Here's how the part is built. I have some questions about the finished solid (model axes, mm). Coordinates: 2 decimals unless noted, no trailing zeros.
```python
from build123d import *

# Parameters (mm, degrees)
BOSS_EXTRUDE1_DEPTH  = 2
CUT_EXTRUDE8_DEPTH   = 3
SKETCH3_R            = 2.15
CUT_EXTRUDE9_DEPTH   = 3
SKETCH4_R            = 12
SKETCH4_R_2          = 1.65
CUT_EXTRUDE10_DEPTH  = 3
SKETCH8_R            = 2.15
CUT_EXTRUDE11_DEPTH  = 3
FILLET1_R            = 1
FILLET1_OF_MIRROR1_R = 1
SKETCH10_R           = 1.65
SKETCH10_R_2         = 1.35
SKETCH10_W           = 40
SKETCH10_H           = 20
CUT_EXTRUDE13_DEPTH  = 3
SKETCH12_R           = 1.65
SKETCH12_W           = 84
SKETCH12_H           = 81
CUT_EXTRUDE15_DEPTH  = 3
FILLET3_R            = 2
SKETCH11_R           = 1.65
CUT_EXTRUDE14_DEPTH  = 3
SKETCH13_R           = 1.65
SKETCH13_R_2         = 1.4
CUT_EXTRUDE16_DEPTH  = 3
SKETCH14_R           = 1.65
CUT_EXTRUDE17_DEPTH  = 3
CUT_EXTRUDE18_DEPTH  = 3


with BuildPart() as part:
    # Sketch1 → Boss-Extrude1 (new body)
    with BuildSketch(Plane(origin=(0, 0, 0), x_dir=(1, 0, 0), z_dir=(0, 1, 0))):
        with BuildLine():
            Line((125, -110), (-125, -110))
            ThreePointArc((-125, -110), (-149.748737342, -99.748737342), (-160, -75))
            Line((-160, -75), (-160, 75))
            ThreePointArc((-160, 75), (-149.748737342, 99.748737342), (-125, 110))
            Line((-125, 110), (125, 110))
            ThreePointArc((125, 110), (149.748737342, 99.748737342), (160, 75))
            Line((160, 75), (160, -75))
            ThreePointArc((160, -75), (149.748737342, -99.748737342), (125, -110))
        make_face()
    extrude(amount=-BOSS_EXTRUDE1_DEPTH)

    # Sketch2 → Cut-Extrude8 (cut, through all)
    with BuildSketch(Plane(origin=(0, 0, 0), x_dir=(1, 0, 0), z_dir=(0, 1, 0))):
        Polygon((100, -70), (100, -14), (113, -14), (113, 3), (137.5, 3), (137.5, -70), align=None)
    cut_extrude8 = extrude(amount=-CUT_EXTRUDE8_DEPTH, mode=Mode.SUBTRACT)

    # Sketch3 → Cut-Extrude9 (cut, through all)
    with BuildSketch(Plane(origin=(0, 0, 0), x_dir=(1, 0, 0), z_dir=(0, 1, 0))):
        with Locations((94.2, -62.670175326)):
            Circle(SKETCH3_R)
        with Locations((107.2, -8.2)):
            Circle(SKETCH3_R)
        with Locations((143.935832446, -30.9314455)):
            Circle(SKETCH3_R)
    cut_extrude9 = extrude(amount=-CUT_EXTRUDE9_DEPTH, mode=Mode.SUBTRACT)

    # Sketch4 → Cut-Extrude10 (cut, through all)
    with BuildSketch(Plane(origin=(0, 0, 0), x_dir=(1, 0, 0), z_dir=(0, 1, 0))):
        with Locations((0, 87)):
            Circle(SKETCH4_R)
        with Locations((-15.5, 87)):
            Circle(SKETCH4_R_2)
        with Locations((15.5, 87)):
            Circle(SKETCH4_R_2)
    extrude(amount=-CUT_EXTRUDE10_DEPTH, mode=Mode.SUBTRACT)

    # Sketch8 → Cut-Extrude11 (cut, through all)
    with BuildSketch(Plane(origin=(0, 0, 0), x_dir=(1, 0, 0), z_dir=(0, 1, 0))):
        with Locations((-132.5, 87.5)):
            Circle(SKETCH8_R)
        with Locations((132.5, 87.5)):
            Circle(SKETCH8_R)
        with Locations((-132.5, -87.5)):
            Circle(SKETCH8_R)
        with Locations((132.5, -87.5)):
            Circle(SKETCH8_R)
    extrude(amount=-CUT_EXTRUDE11_DEPTH, mode=Mode.SUBTRACT)

    # Fillet1
    fillet1_edges = [part.edges().sort_by_distance(p)[0] for p in [
        (137.5, -1, 70),
        (100, -1, 70),
        (100, -1, 14),
        (113, -1, 14),
        (113, -1, -3),
        (137.5, -1, -3),
    ]]
    fillet(fillet1_edges, radius=FILLET1_R)

    # Mirror1: Cut-Extrude8, Cut-Extrude9 across plane
    add(cut_extrude8.mirror(Plane(origin=(0, 0, 0), x_dir=(0, 0, 1), z_dir=(1, 0, 0))), mode=Mode.SUBTRACT)
    add(cut_extrude9.mirror(Plane(origin=(0, 0, 0), x_dir=(0, 0, 1), z_dir=(1, 0, 0))), mode=Mode.SUBTRACT)

    # Fillet1 of Mirror1
    fillet1_of_mirror1_edges = [part.edges().sort_by_distance(p)[0] for p in [
        (-137.5, -1, 70),
        (-100, -1, 70),
        (-100, -1, 14),
        (-113, -1, 14),
        (-113, -1, -3),
        (-137.5, -1, -3),
    ]]
    fillet(fillet1_of_mirror1_edges, radius=FILLET1_OF_MIRROR1_R)

    # Sketch10 → Cut-Extrude13 (cut, through all)
    with BuildSketch(Plane(origin=(0, 0, 0), x_dir=(1, 0, 0), z_dir=(0, 1, 0))):
        with Locations((18.35, -43)):
            Circle(SKETCH10_R)
        with Locations((-18.35, -43)):
            Circle(SKETCH10_R)
        with Locations((-18.35, -79.7)):
            Circle(SKETCH10_R)
        with Locations((18.35, -79.7)):
            Circle(SKETCH10_R)
        with Locations((-56, 67.5)):
            Circle(SKETCH10_R_2)
        with Locations((-114, 67.5)):
            Circle(SKETCH10_R_2)
        with Locations((-114, 18.5)):
            Circle(SKETCH10_R_2)
        with Locations((-56, 18.5)):
            Circle(SKETCH10_R_2)
        with Locations((-7.5, -34.9314455)):
            Circle(SKETCH10_R)
        with Locations((7.5, -34.9314455)):
            Circle(SKETCH10_R)
        with Locations((-35, 43)):
            Rectangle(SKETCH10_W, SKETCH10_H)
    extrude(amount=-CUT_EXTRUDE13_DEPTH, mode=Mode.SUBTRACT)

    # Sketch12 → Cut-Extrude15 (cut, through all)
    with BuildSketch(Plane(origin=(0, 0, 0), x_dir=(1, 0, 0), z_dir=(0, 1, 0))):
        with Locations((-42, 68.5)):
            Circle(SKETCH12_R)
        with Locations((52, 68.5)):
            Circle(SKETCH12_R)
        with Locations((-42, -22.5)):
            Circle(SKETCH12_R)
        with Locations((52, -22.5)):
            Circle(SKETCH12_R)
        with Locations((5, 23)):
            Rectangle(SKETCH12_W, SKETCH12_H)
    extrude(amount=-CUT_EXTRUDE15_DEPTH, mode=Mode.SUBTRACT)

    # Fillet3
    fillet3_edges = [part.edges().sort_by_distance(p)[0] for p in [
        (-55, -1, -33),
        (-55, -1, -53),
        (-37, -1, -53),
        (-37, -1, -33),
        (-37, -1, 17.5),
        (-37, -1, -63.5),
        (47, -1, -63.5),
        (47, -1, 17.5),
    ]]
    fillet(fillet3_edges, radius=FILLET3_R)

    # Sketch11 → Cut-Extrude14 (cut, through all)
    with BuildSketch(Plane(origin=(0, 0, 0), x_dir=(1, 0, 0), z_dir=(0, 1, 0))):
        with Locations((90, 65)):
            Circle(SKETCH11_R)
        with Locations((140, 65)):
            Circle(SKETCH11_R)
        with Locations((90, 15)):
            Circle(SKETCH11_R)
        with Locations((140, 15)):
            Circle(SKETCH11_R)
        with Locations((-65, -20)):
            Circle(SKETCH11_R)
    extrude(amount=-CUT_EXTRUDE14_DEPTH, mode=Mode.SUBTRACT)

    # Sketch13 → Cut-Extrude16 (cut, through all)
    with BuildSketch(Plane(origin=(0, 0, 0), x_dir=(1, 0, 0), z_dir=(0, 1, 0))):
        with Locations((-47.25, 90)):
            Circle(SKETCH13_R)
        with Locations((47.25, 90)):
            Circle(SKETCH13_R)
        with Locations((-43, 95)):
            Circle(SKETCH13_R_2)
        with Locations((43, 95)):
            Circle(SKETCH13_R_2)
    extrude(amount=-CUT_EXTRUDE16_DEPTH, mode=Mode.SUBTRACT)

    # Sketch14 → Cut-Extrude17 (cut, through all)
    with BuildSketch(Plane(origin=(0, 0, 0), x_dir=(1, 0, 0), z_dir=(0, 1, 0))):
        with Locations((30, -51.35)):
            Circle(SKETCH14_R)
        with Locations((30, -71.35)):
            Circle(SKETCH14_R)
    cut_extrude17 = extrude(amount=-CUT_EXTRUDE17_DEPTH, mode=Mode.SUBTRACT)

    # Mirror2: Cut-Extrude17 across plane
    add(cut_extrude17.mirror(Plane(origin=(0, 0, 0), x_dir=(0, 0, 1), z_dir=(1, 0, 0))), mode=Mode.SUBTRACT)

    # Sketch16 → Cut-Extrude18 (cut, through all)
    with BuildSketch(Plane(origin=(0, 0, 0), x_dir=(1, 0, 0), z_dir=(0, 1, 0))):
        with BuildLine():
            Line((59.5, 70), (59.5, 76))
            ThreePointArc((59.5, 76), (61, 77.5), (62.5, 76))
            Line((62.5, 76), (62.5, 70))
            ThreePointArc((62.5, 70), (61, 68.5), (59.5, 70))
        make_face()
        with BuildLine():
            Line((67.5, 70), (67.5, 76))
            ThreePointArc((67.5, 76), (69, 77.5), (70.5, 76))
            Line((70.5, 76), (70.5, 70))
            ThreePointArc((70.5, 70), (69, 68.5), (67.5, 70))
        make_face()
        with BuildLine():
            Line((59.5, -30), (59.5, -24))
            ThreePointArc((59.5, -24), (61, -22.5), (62.5, -24))
            Line((62.5, -24), (62.5, -30))
            ThreePointArc((62.5, -30), (61, -31.5), (59.5, -30))
        make_face()
        with BuildLine():
            Line((67.5, -30), (67.5, -24))
            ThreePointArc((67.5, -24), (69, -22.5), (70.5, -24))
            Line((70.5, -24), (70.5, -30))
            ThreePointArc((70.5, -30), (69, -31.5), (67.5, -30))
        make_face()
    extrude(amount=-CUT_EXTRUDE18_DEPTH, mode=Mode.SUBTRACT)


solid = part.part
```
1. We'd pull the mould along Z, two halves only. Please class faces 1 (the cylindrical face through (-149.475, -0.986, 100.019)), 2 (the flat face through (2, -2, 23)), 3 (the cylindrical face through (-2.601, -0.986, -75.285)): +Z half, -Z half, draft (parallel to the pull), parting line (faces both ways), or undercut.
2. I need wall thicknesses on line 1 along Z through (x, y) = (29.5, -1.7); line 2 along Z through (x, y) = (-30, -1.2); line 3 along X through (y, z) = (-1.25, 4.5). Which ranges of each line are inside material? Lowest first, please.
3. For pin 1 (8 mm diameter, centred on x = 119, z = 1.5, fed in from +Y); pin 2 (1 mm diameter, centred on x = 130, y = -1, fed in from +Z), each with a flat end and sliding along its axis, tell me the tip position at first contact or that it passes through.
4. I want a section at A-A (y = -0.45). Give the number of separate pieces and of enclosed holes in the cut face, then the cut area to 3 significant figures.
Response values:
1. face 1: +Z half
1. face 2: draft
1. face 3: undercut
2. line 1: z = -110 to -63.5, 17.5 to 49.78, 52.92 to 69.78, 72.92 to 110
2. line 2: z = -110 to -63.5, 17.5 to 49.7, 53 to 69.7, 73 to 110
2. line 3: x = -160 to -137.5, -113 to -37, 47 to 113, 137.5 to 160
3. pin 1: passes through
3. pin 2: stops at z = 109.71
4. separate pieces: 1
4. enclosed holes: 47
4. area: 56,200 mm2
